Build history of the part. All positions in model axes, mm. A direction names the side the tool comes from. Round coordinates to 2 decimals unless told otherwise and drop trailing zeros. Write each loop counter-clockwise with the first axis right and the second up, starting at its lowest first coordinate (ties: lowest second). Pieces come first, ordered by that corner, then holes. Notation, with made-up numbers: (16, 40) - (29, 40) arc R15 cw to (29, 54) - close; hole circle Ø3 at (84, 66.5). An arc over 180 degrees is marked (long way). Answer as a JSON object with one key per item and string values. Group by question number.
Item 1: Slice it at A-A, the plane z = 62.5. Give the number of separate pieces and of enclosed holes in the cut face, then the cut area to 3 significant figures.
Item 2: Which spindle directions (+Z, -Z, +X, -X, +Y, -Y) get a long thin tool onto all of the face, cutting with end or side? Do faces 5 (the flat face through (53, 3, -53)), 6 (the flat face through (53, 22, 53)), 7 (the cylindrical face through (68.335, 12.633, 15.175)), 8 (the flat face through (-53, 3, 53)). Say none if no direction does.
Item 3: Probe line 1 (Y direction, x = -55, z = 54); line 2 (X direction, y = 21.5, z = 26.5); line 3 (X direction, y = 9, z = -11). List the from-to ranges inside material, lowest first. Write a range as from..to.
Item 4: Slice it at C-C, the plane x = 31. List the corners of the cut face in (y, z).
Item 5: Flat gauge pins, fed straight in: pin 1 (1 mm diameter, centred on x = 8, y = 11.5, fed in from -Z); pin 2 (2.5 mm diameter, centred on x = -62.5, z = 62.5, fed in from -Y); pin 3 (10 mm diameter, centred on y = 12, z = -47.5, fed in from -X); pin 4 (10 mm diameter, centred on y = 8.5, z = 49.5, fed in from -X). Where does each tip first touch, or does it go through?
Item 6: Slice it at B-B, the plane z = -22. List the corners of the cut face in (x, y), then the cut area to 3 significant figures.
Item 7: Two-plate mould, pull along X, no slides. Class faces 1 (the flat face through (70, 24, 1)), 2 (the cylindrical face through (-64.286, 1.479, -61.131)), 3 (the flat face through (-37, 0, -57)), 4 (the cylindrical face through (-64.286, 23.479, -61.131)): +X half, -X half, draft (parallel to the pull), parting line (faces both ways), or undercut.
from build123d import *

# Parameters (mm, degrees)
SKETCH2_OUTSIDE_W            = 258.79
SKETCH2_OUTSIDE_H            = 258.79
SKETCH2_OUTSIDE_W_2          = 140
SKETCH2_OUTSIDE_H_2          = 140
SQUARE_SHAPE_CUTOUT_DEPTH    = 144.614066163
M4_CLEARANCE_HOLE1_OUTLINE_R = 2.25
M4_CLEARANCE_HOLE1_DEPTH     = 25


# Read off the part's stored shape, not the designer's step: M4 Clearance Hole1
with BuildPart() as part:
    # Sketch1 → body (revolve)
    with BuildSketch(Plane.XY, mode=Mode.PRIVATE) as body_sk:
        Polygon((67, 0), (100, 0), (100, 3), (70, 3), (70, 22), (100, 22), (100, 25), (67, 25), align=None)
    revolve(body_sk.sketch.rotate(Axis((0, 0, 0), (0, 1, 0)), 90), axis=Axis((0, 0, 0), (0, 1, 0)))

    # Sketch2 outside → square_shape_cutout (cut, through all)
    with BuildSketch(Plane(origin=(0, 25, 0), x_dir=(1, 0, 0), z_dir=(0, 1, 0))):
        Rectangle(SKETCH2_OUTSIDE_W, SKETCH2_OUTSIDE_H)
        Rectangle(SKETCH2_OUTSIDE_W_2, SKETCH2_OUTSIDE_H_2, mode=Mode.SUBTRACT)
    extrude(amount=-SQUARE_SHAPE_CUTOUT_DEPTH, mode=Mode.SUBTRACT)

    # M4 Clearance Hole1 outline → M4 Clearance Hole1 (cut)
    with BuildSketch(Plane(origin=(0, 0, 0), x_dir=(1, 0, 0), z_dir=(0, 1, 0))):
        with Locations((62.5, 62.5)):
            Circle(M4_CLEARANCE_HOLE1_OUTLINE_R)
        with Locations((-62.5, -62.5)):
            Circle(M4_CLEARANCE_HOLE1_OUTLINE_R)
        with Locations((62.5, -62.5)):
            Circle(M4_CLEARANCE_HOLE1_OUTLINE_R)
        with Locations((-62.5, 62.5)):
            Circle(M4_CLEARANCE_HOLE1_OUTLINE_R)
    extrude(amount=M4_CLEARANCE_HOLE1_DEPTH, mode=Mode.SUBTRACT)


solid = part.part
Geometry says:
{
 "1": {"separate pieces": "6", "enclosed holes": "0", "area": "777 mm^2"},
 "2": {"face 5": "-Z, +X", "face 6": "+Z, +X", "face 7": "none", "face 8": "+Z, -X"},
 "3": {"line 1": "y = 0..3, 22..25", "line 2": "x = -64.79..-61.54, 61.54..64.79", "line 3": "x = -69.13..-66.09, 66.09..69.13"},
 "4": {"outline": "(0, -70) - (3, -70) - (3, -62.76) - (22, -62.76) - (22, -70) - (25, -70) - (25, -59.4) - (0, -59.4) - close; (0, 59.4) - (25, 59.4) - (25, 70) - (22, 70) - (22, 62.76) - (3, 62.76) - (3, 70) - (0, 70) - close"},
 "5": {"pin 1": "stops at z = -69.6", "pin 2": "passes through", "pin 3": "stops at x = -55.62", "pin 4": "stops at x = -54.03"},
 "6": {"outline": "(-70, 0) - (-63.29, 0) - (-63.29, 25) - (-70, 25) - (-70, 22) - (-66.45, 22) - (-66.45, 3) - (-70, 3) - close; (63.29, 0) - (70, 0) - (70, 3) - (66.45, 3) - (66.45, 22) - (70, 22) - (70, 25) - (63.29, 25) - close", "area": "201 mm^2"},
 "7": {"face 1": "+X half", "face 2": "undercut", "face 3": "draft", "face 4": "undercut"}
}
